The listing builds one solid part. Answer for the finished solid, in the listing's coordinates (mm). A direction names the side the tool comes from. Coordinates: 2 decimals unless noted, no trailing zeros. Write each loop counter-clockwise with the first axis right and the second up, starting at its lowest first coordinate (ties: lowest second). Pieces come first, ordered by that corner, then holes.
(1) The part is cut by section D-D on x = -16. Determine the outline of the cut face in (y, z).
(2) The part is cut by section B-B on z = 0. Determine the outline of the cut face in (x, y).
(3) Given P1, Ø4, axis at x = 18.5, z = 8.5, coming from the +Y side; P2, Ø1.5, axis at y = 16.5, z = 16.5, coming from the +X side, each flat-ended and moving along its own axis, determine where each tip first touches the part or whether it passes through.
(4) Straight lines are drawn through the part: line 1 (Y direction, x = -24.6, z = 0); line 2 (Y direction, x = 8, z = -6); line 3 (X direction, y = 39.5, z = -8). For each, find the intervals that lie inside material, in ascending order.
(5) For a pull along Y with two mould halves and no side action, classify faces 1 (the cylindrical face through (-25.52, 19.76, -2.38)), 2 (the flat face through (-26, 51.75, 0)), 3 (the flat face through (-12.1, 2.8, -25)) as +Y half, -Y half, draft (parallel to the pull), parting line (faces both ways), or undercut.
(6) Which of the six approach directions +Z, -Z, +X, -X, +Y, -Y give full straight-line access (tool end or side, diameter ignored) to faces 4 (the flat face through (1, 3, 0)), 5 (the flat face through (-27, 20, 6))?
(7) The part is cut by section C-C on z = 15.5. Determine the outline of the cut face in (x, y).
(8) The part is cut by section A-A on y = 30.5. Determine the outline of the cut face in (x, z).
from build123d import *

# Parameters (mm, degrees)
SKETCH1_W           = 54
SKETCH1_H           = 50
BOSS_EXTRUDE1_DEPTH = 3
SKETCH2_W           = 3
SKETCH2_H           = 50
BOSS_EXTRUDE2_DEPTH = 48.75
SKETCH3_R           = 11
CUT_EXTRUDE1_DEPTH  = 55


with BuildPart() as part:
    # Sketch1 → Boss-Extrude1 (new body)
    with BuildSketch(Plane(origin=(0, 0, 0), x_dir=(1, 0, 0), z_dir=(0, 1, 0))):
        Rectangle(SKETCH1_W, SKETCH1_H)
    extrude(amount=BOSS_EXTRUDE1_DEPTH)

    # Sketch2 → Boss-Extrude2 (add)
    with BuildSketch(Plane(origin=(0, 3, 0), x_dir=(1, 0, 0), z_dir=(0, 1, 0))):
        with Locations((-25.5, 0)):
            Rectangle(SKETCH2_W, SKETCH2_H)
    extrude(amount=BOSS_EXTRUDE2_DEPTH)

    # Sketch3 → Cut-Extrude1 (cut, through all)
    with BuildSketch(Plane.ZY.offset(27)):
        with Locations((0, 30.5)):
            Circle(SKETCH3_R)
    extrude(amount=-CUT_EXTRUDE1_DEPTH, mode=Mode.SUBTRACT)


solid = part.part
Model answer:
1. outline: (0, -25) - (3, -25) - (3, 25) - (0, 25) - close
2. outline: (-27, 0) - (27, 0) - (27, 3) - (-24, 3) - (-24, 19.5) - (-27, 19.5) - close; (-27, 41.5) - (-24, 41.5) - (-24, 51.75) - (-27, 51.75) - close
3. P1: stops at y = 3
3. P2: stops at x = -24
4. line 1: y = 0 to 19.5, 41.5 to 51.75
4. line 2: y = 0 to 3
4. line 3: x = -27 to -24
5. face 1: undercut
5. face 2: +Y half
5. face 3: draft
6. face 4: +Z, -Z, +X, +Y
6. face 5: +Z, -Z, -X, +Y, -Y
7. outline: (-27, 0) - (27, 0) - (27, 3) - (-24, 3) - (-24, 51.75) - (-27, 51.75) - close
8. outline: (-27, -25) - (-24, -25) - (-24, -11) - (-27, -11) - close; (-27, 11) - (-24, 11) - (-24, 25) - (-27, 25) - close
